Autodesk Inventor part; units mm, degrees
ref_plane "YZ Plane" through (0, 0, 0) normal (1, 0, 0) x (0, 1, 0)
ref_plane "XZ Plane" through (0, 0, 0) normal (0, 1, 0) x (-1, 0, 0)
ref_plane "XY Plane" through (0, 0, 0) normal (0, 0, 1) x (1, 0, 0)
sketch "Sketch1" plane through (0, 0, 0) normal (0, 1, 0) x (-1, 0, 0)
  circle A0 centre (0, -18.35) radius 2.5
  circle A1 centre (0, 18.35) radius 2.5
  circle A2 centre (0, 0) radius 4
  circle A3 centre (0, 0) radius 5.8
  circle A4 centre (0, 0) radius 12.75
  line L0 (4.9784, -20.6879) -> (12.0386, -5.6534)
  line L1 (-4.9784, -20.6879) -> (-12.0386, -5.6534)
  line L2 (4.9784, 20.6879) -> (12.0386, 5.6534)
  line L3 (-4.9784, 20.6879) -> (-12.0386, 5.6534)
  arc A5 (-4.9784, -20.6879) -> (4.9784, -20.6879) centre (0, -18.35) ccw
  arc A6 (4.9784, 20.6879) -> (-4.9784, 20.6879) centre (0, 18.35) ccw
  arc A7 (-12.0386, 5.6534) -> (-12.0386, -5.6534) centre (0, 0) ccw
  arc A8 (12.0386, -5.6534) -> (12.0386, 5.6534) centre (0, 0) ccw
  dimension "d2" = 18.35
  dimension "d4" = 18.35
  dimension "d5" = 5
  dimension "d6" = 5
  dimension "d7" = 8
  dimension "d8" = 11.6
  dimension "d9" = 25.5
  dimension "d10" = 0
  dimension "d12" = 0
extrude "Extrusion1" add sketch "Sketch1" along normal blind 11.1 contours A3
sketch "Sketch2" plane through (0, 0, 0) normal (0, -1, 0) x (1, 0, 0)
  circle A0 centre (0, -18.35) radius 2.5
  circle A1 centre (0, 18.35) radius 2.5
  circle A2 centre (0, 0) radius 4
  circle A3 centre (0, 0) radius 5.8
  circle A4 centre (0, 0) radius 12.75
  line L0 (4.9784, -20.6879) -> (12.0386, -5.6534)
  line L1 (-4.9784, -20.6879) -> (-12.0386, -5.6534)
  line L2 (4.9784, 20.6879) -> (12.0386, 5.6534)
  line L3 (-4.9784, 20.6879) -> (-12.0386, 5.6534)
  arc A5 (-4.9784, -20.6879) -> (4.9784, -20.6879) centre (0, -18.35) ccw
  arc A6 (4.9784, 20.6879) -> (-4.9784, 20.6879) centre (0, 18.35) ccw
  arc A7 (-12.0386, 5.6534) -> (-12.0386, -5.6534) centre (0, 0) ccw
  arc A8 (12.0386, -5.6534) -> (12.0386, 5.6534) centre (0, 0) ccw
  dimension "d15" = 18.35
  dimension "d16" = 18.35
  dimension "d17" = 5
  dimension "d18" = 5
  dimension "d19" = 8
  dimension "d20" = 11.6
  dimension "d21" = 25.5
  dimension "d22" = 0
  dimension "d23" = 0
  dimension "d24" = 0
  dimension "d25" = 0
extrude "Extrusion2" add sketch "Sketch2" against normal blind 8 contours A4
sketch "Sketch3" plane through (0, 0, 0) normal (0, -1, 0) x (1, 0, 0)
  circle A0 centre (0, -18.35) radius 2.5
  circle A1 centre (0, 18.35) radius 2.5
  circle A2 centre (0, 0) radius 4
  line L0 (4.9784, -20.6879) -> (12.0386, -5.6534)
  line L1 (-4.9784, -20.6879) -> (-12.0386, -5.6534)
  line L2 (4.9784, 20.6879) -> (12.0386, 5.6534)
  line L3 (-4.9784, 20.6879) -> (-12.0386, 5.6534)
  arc A3 (-4.9784, -20.6879) -> (4.9784, -20.6879) centre (0, -18.35) ccw
  arc A4 (4.9784, 20.6879) -> (-4.9784, 20.6879) centre (0, 18.35) ccw
  arc A5 (-12.0386, 5.6534) -> (-12.0386, -5.6534) centre (0, 0) ccw
  arc A6 (12.0386, -5.6534) -> (12.0386, 5.6534) centre (0, 0) ccw
  dimension "d28" = 18.35
  dimension "d29" = 18.35
  dimension "d30" = 5
  dimension "d31" = 5
  dimension "d32" = 8
  dimension "d35" = 0
  dimension "d36" = 0
  dimension "d37" = 0
  dimension "d38" = 0
extrude "Extrusion3" add sketch "Sketch3" against normal blind 4
ref_plane "Work Plane1" through (0, 4, 23.85) normal (1, 0, 0) x (0, -1, 0)
properties part number "Bearing"
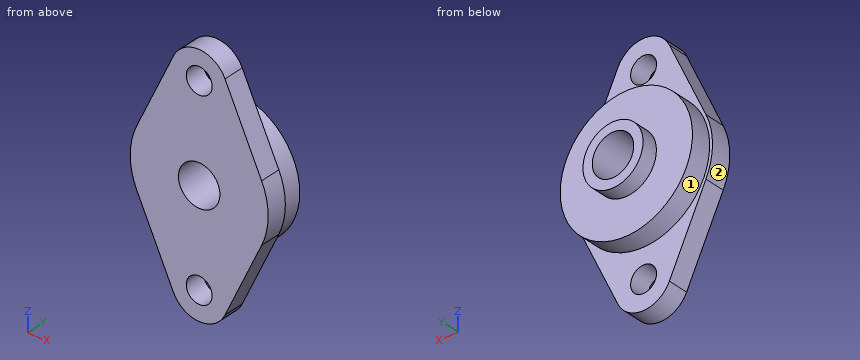
Source: CAD feature listing. Evaluate the final solid. Frame: model axes, mm. Face numbers are marked on the shaded views. A direction names the side the tool comes from. Give positions to 0.01 mm unless a question says otherwise; leave off trailing zeros. Write each loop counter-clockwise with the first axis right and the second up, starting at its lowest first coordinate (ties: lowest second). Pieces come first, ordered by that corner, then holes. Notation, with made-up numbers: (7.25, 63) - (15.25, 63) arc R23 ccw to (15.25, 96) - close; hole circle Ø1 at (46, 21.25). An arc over 180 degrees is marked (long way). Write item = value, one per line. Start each with the question number.
Q1. Cut plane C-C, the plane y = 3.25. Return loops of the section in (x, z).
Q2. Cut plane B-B, the plane x = 0. Return loops of the section in (y, z), then the cut area to 3 significant figures.
Q3. Material intervals for probe 1 along Y at (x, z) = (3.25, 17.5); probe 2 along Y at (x, z) = (7, -2); probe 3 along X at (y, z) = (3, -0.5), sorted ascending.
Q4. Reachability of the marked faces 1 and 2 from +Z, -Z, +X, -X, +Y, -Y: full face, straight path, thin tool, end or side. Return the list, or none.
Q5. Cut plane A-A, the plane z = 0. Return loops of the section in (x, y).
Q6. Cut plane D-D, the plane z = 17.5. Return loops of the section in (x, y), then the cut area to 3 significant figures.
Q7. Pin query (flat end, axial travel): pin 1 Ø6 at (y, z) = (3, -16.5) entering from +X; pin 2 Ø2 at (y, z) = (1, 17) entering from +X; pin 3 Ø1.5 at (x, z) = (-7.5, -4) entering from +Y; pin 4 Ø6.5 at (x, z) = (0, 0) entering from -Y. Return the tip coordinate at first contact, or that it passes through.
Computed values:
q1.outline = (-12.04, -5.65) - (-4.98, -20.69) arc R5.5 ccw to (4.98, -20.69) - (12.04, -5.65) arc R13.3 ccw to (12.04, 5.65) - (4.98, 20.69) arc R5.5 ccw to (-4.98, 20.69) - (-12.04, 5.65) arc R13.3 ccw to start; hole circle Ø8 at (0, 0); hole circle Ø5 at (0, -18.35); hole circle Ø5 at (0, 18.35)
q2.outline = (0, -23.85) - (4, -23.85) - (4, -20.85) - (0, -20.85) - close; (0, -15.85) - (4, -15.85) - (4, -12.75) - (8, -12.75) - (8, -5.8) - (11.1, -5.8) - (11.1, -4) - (0, -4) - close; (0, 4) - (11.1, 4) - (11.1, 5.8) - (8, 5.8) - (8, 12.75) - (4, 12.75) - (4, 15.85) - (0, 15.85) - close; (0, 20.85) - (4, 20.85) - (4, 23.85) - (0, 23.85) - close
q2.area = 200 mm²
q3.probe_1 = 0 to 4
q3.probe_2 = 0 to 8
q3.probe_3 = -13.29 to -3.97, 3.97 to 13.29
q4.face_1 = +Y
q4.face_2 = -X, +Y, -Y
q5.outline = (-13.3, 0) - (-4, 0) - (-4, 11.1) - (-5.8, 11.1) - (-5.8, 8) - (-12.75, 8) - (-12.75, 4) - (-13.3, 4) - close; (4, 0) - (13.3, 0) - (13.3, 4) - (12.75, 4) - (12.75, 8) - (5.8, 8) - (5.8, 11.1) - (4, 11.1) - close
q6.outline = (-6.48, 0) - (-2.35, 0) - (-2.35, 4) - (-6.48, 4) - close; (2.35, 0) - (6.48, 0) - (6.48, 4) - (2.35, 4) - close
q6.area = 33.0 mm²
q7.pin_1 = 8.35
q7.pin_2 = 7.18
q7.pin_3 = 8
q7.pin_4 = through
